The model under review builds one solid part; all positions refer to its coordinate system, in mm. Give positions to 0.01 mm unless a question says otherwise; leave off trailing zeros. Write each loop counter-clockwise with the first axis right and the second up, starting at its lowest first coordinate (ties: lowest second). Pieces come first, ordered by that corner, then holes. Notation, with made-up numbers: (-8.75, 35) -> (9.25, 35) arc R17 cw to (9.25, 48) -> close; hole circle Ø7 at (-1, 34.5). An arc over 180 degrees is marked (long way). Use CSV: the item, a comma, the result in double quotes.
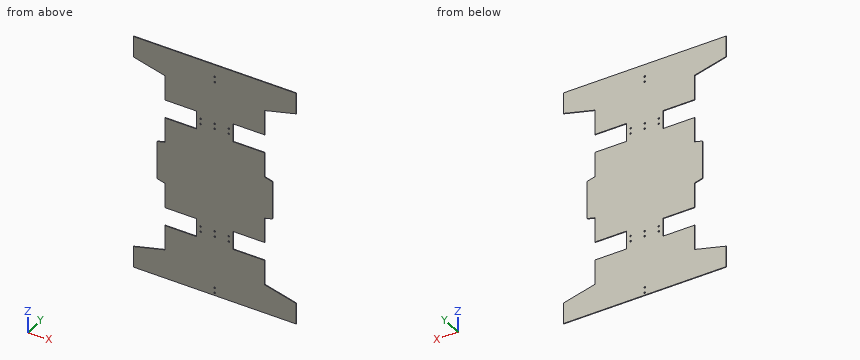
Autodesk Inventor part; units mm, degrees
ref_plane "YZ Plane" through (0, 0, 0) normal (1, 0, 0) x (0, 1, 0)
ref_plane "XZ Plane" through (0, 0, 0) normal (0, 1, 0) x (-1, 0, 0)
ref_plane "XY Plane" through (0, 0, 0) normal (0, 0, 1) x (1, 0, 0)
sketch "Sketch1" plane through (0, 0, 0) normal (0, 1, 0) x (-1, 0, 0)
  line L0 (359.9997, -324.9998) -> (359.9997, -389.9998)
  line L1 (359.9997, -389.9998) -> (239.9998, -420.0002)
  line L2 (359.9997, -194.9998) -> (359.9997, -129.9998)
  line L3 (359.9997, -129.9998) -> (239.9997, -99.9998)
  line L4 (359.9998, -615.0001) -> (359.9998, -550.0001)
  line L5 (359.9998, -550.0001) -> (239.9998, -520.0001)
  line L6 (359.9998, -745.0001) -> (359.9998, -810.0001)
  line L7 (359.9998, -810.0001) -> (239.9998, -840.0001)
  line L8 (740, -325.0005) -> (740, -390.0005)
  line L9 (740, -390.0005) -> (860, -420.0005)
  line L10 (740, -195.0005) -> (740, -130.0005)
  line L11 (740, -130.0005) -> (860, -100.0005)
  line L12 (740, -615.0001) -> (740, -550.0005)
  line L13 (740, -550.0005) -> (860, -520.0005)
  line L14 (740, -744.9998) -> (740, -809.9998)
  line L15 (740, -809.9998) -> (860, -839.9998)
  line L16 (860, -100.0005) -> (860, -19.9997)
  line L17 (860, -839.9998) -> (860, -919.9998)
  line L18 (239.9997, -99.9998) -> (239.9997, -19.9997)
  line L19 (239.9998, -840.0001) -> (239.9998, -920.0001)
  line L20 (859.9998, -19.9997) -> (379.9998, -19.9997)
  line L21 (860, -19.9997) -> (379.9998, -19.9997)
  line L22 (479.9997, -19.9997) -> (239.9997, -19.9997)
  line L23 (860, -919.9998) -> (139.9998, -919.9998)
  line L24 (239.9997, -19.9997) -> (859.9998, -19.9997)
  line L25 (860, -520.0005) -> (860, -420.0005)
  line L26 (239.9998, -520.0001) -> (239.9998, -420.0002)
  line L27 (479.9998, -744.9997) -> (479.9998, -745.0001)
  line L28 (479.9998, -745.0001) -> (479.9998, -615.0001)
  line L29 (479.9998, -615.0001) -> (359.9998, -615.0001)
  line L30 (479.9998, -745.0001) -> (359.9998, -745.0001)
  line L31 (620, -679.9998) -> (620, -745.0001)
  line L32 (620, -745.0001) -> (740, -744.9998)
  line L33 (620, -679.9998) -> (620, -615.0001)
  line L34 (740, -615.0001) -> (620, -615.0001)
  line L35 (620, -260.0005) -> (620, -325.0005)
  line L36 (620, -325.0005) -> (620, -195.0005)
  line L37 (620, -195.0005) -> (740, -195.0005)
  line L38 (620, -325.0005) -> (740, -325.0005)
  line L39 (479.9997, -260.0005) -> (479.9993, -325.0005)
  line L40 (479.9993, -325.0005) -> (359.9997, -324.9998)
  line L41 (479.9997, -260.0005) -> (479.9997, -195.0005)
  line L42 (479.9997, -195.0005) -> (359.9997, -194.9998)
  point P0 (479.9997, -19.9997)
  point P1 (740, -810.0001)
  point P2 (740, -550.0001)
  point P3 (740, -390.0001)
  point P4 (740, -130.0001)
  point P5 (239.9998, -919.9998)
  point P6 (239.9998, -919.9998)
  dimension "d44" = 0.45
  dimension "d16" = 80
  dimension "d23" = 65
extrude "Extrusion1" add sketch "Sketch1" along normal blind 3
sketch "Sketch2" plane through (0, 3, 0) normal (0, 1, 0) x (1, 0, 0)
  line L0 (-620, 325.0005) -> (-620, 195.0005)
  line L1 (-620, 260.0005) -> (-620, 225.0005)
  line L2 (-620, 225.0005) -> (-740, 225.0005)
  line L3 (-740, 195.0005) -> (-740, 130.0005)
  line L4 (-740, 225.0005) -> (-740, 195.0005)
  line L5 (-620, 260.0005) -> (-620, 295.0005)
  line L6 (-620, 295.0005) -> (-740, 295.0005)
  line L7 (-740, 295.0005) -> (-740, 325.0005)
  line L8 (-740, 325.0005) -> (-620, 325.0005)
  line L9 (-740, 325.0005) -> (-620, 325.0005)
  line L10 (-620, 325.0005) -> (-620, 295.0005)
  line L11 (-620, 225.0005) -> (-620, 195.0005)
  line L12 (-620, 195.0005) -> (-740, 195.0005)
  line L13 (-479.9997, 195.0005) -> (-479.9997, 260.0005)
  line L14 (-359.9997, 194.9998) -> (-479.9997, 195.0005)
  line L15 (-479.9997, 195.0005) -> (-359.9997, 194.9998)
  line L16 (-359.9997, 194.9998) -> (-359.9995, 225.0005)
  line L17 (-359.9995, 225.0005) -> (-479.9995, 225.0012)
  line L18 (-479.9995, 225.0012) -> (-479.9995, 295.0005)
  line L19 (-479.9997, 260.0005) -> (-479.9993, 325.0005)
  line L20 (-479.9993, 325.0005) -> (-359.9997, 324.9998)
  line L21 (-479.9993, 325.0005) -> (-359.9997, 324.9998)
  line L22 (-359.9997, 324.9998) -> (-359.9991, 295.0005)
  line L23 (-479.9995, 295.0005) -> (-359.9991, 295.0005)
  line L24 (-620, 745.0001) -> (-620, 615.0001)
  line L25 (-620, 680.0001) -> (-620, 645.0001)
  line L26 (-620, 645.0001) -> (-740, 645.0001)
  line L27 (-740, 645.0001) -> (-740, 615.0001)
  line L28 (-740, 615.0001) -> (-620, 615.0001)
  line L29 (-620, 615.0001) -> (-620, 645.0001)
  line L30 (-620, 680.0001) -> (-620, 715.0001)
  line L31 (-620, 715.0001) -> (-740, 715.0001)
  line L32 (-740, 744.9998) -> (-620, 745.0001)
  line L33 (-740, 715.0001) -> (-740, 744.9998)
  line L34 (-740, 744.9998) -> (-620, 745.0001)
  line L35 (-620, 745.0001) -> (-620, 715.0001)
  line L36 (-479.9998, 615.0001) -> (-479.9998, 745.0001)
  line L37 (-479.9998, 680.0001) -> (-479.9998, 645.0001)
  line L38 (-479.9998, 645.0001) -> (-359.9998, 645.0001)
  line L39 (-359.9998, 615.0001) -> (-479.9998, 615.0001)
  line L40 (-359.9998, 645.0001) -> (-359.9998, 615.0001)
  line L41 (-359.9998, 615.0001) -> (-479.9998, 615.0001)
  line L42 (-479.9998, 615.0001) -> (-479.9998, 645.0001)
  line L43 (-479.9998, 680.0001) -> (-479.9998, 715.0001)
  line L44 (-479.9998, 715.0001) -> (-359.9998, 715.0001)
  line L45 (-479.9998, 745.0001) -> (-359.9998, 745.0001)
  line L46 (-359.9998, 715.0001) -> (-359.9998, 745.0001)
  line L47 (-359.9998, 745.0001) -> (-479.9998, 745.0001)
  line L48 (-479.9998, 745.0001) -> (-479.9998, 715.0001)
  point P0 (0, 0)
  dimension "d26" = 35
  dimension "d27" = 35
  dimension "d28" = 35
  dimension "d29" = 35
  dimension "d30" = 35
  dimension "d31" = 35
extrude "Extrusion2" add sketch "Sketch2" against normal up to surface (3 mm away)
sketch "Sketch3" plane through (0, 3, 0) normal (0, 1, 0) x (1, 0, 0)
  line L0 (-620, 295.0005) -> (-620, 225.0005)
  line L1 (-620, 260.0005) -> (-620, 240.0005)
  line L2 (-620, 240.0005) -> (-479.9995, 240.0005)
  line L3 (-479.9995, 225.0012) -> (-479.9995, 295.0005)
  line L4 (-479.9995, 240.0005) -> (-479.9995, 280.0005)
  line L5 (-479.9995, 280.0005) -> (-620, 280.0005)
  line L6 (-620, 280.0005) -> (-620, 260.0005)
  line L7 (-620, 715.0001) -> (-620, 645.0001)
  line L8 (-620, 680.0001) -> (-620, 660.0001)
  line L9 (-620, 660.0001) -> (-479.9998, 660.0001)
  line L10 (-479.9998, 645.0001) -> (-479.9998, 715.0001)
  line L11 (-479.9998, 660.0001) -> (-479.9998, 680.0001)
  line L12 (-479.9998, 680.0001) -> (-479.9998, 700.0001)
  line L13 (-479.9998, 700.0001) -> (-620, 700.0001)
  line L14 (-620, 700.0001) -> (-620, 680.0001)
  point P0 (0, 0)
  dimension "d34" = 20
  dimension "d35" = 40
  dimension "d36" = 20
  dimension "d37" = 20
  dimension "d38" = 20
sketch "Sketch4" plane through (0, 3, 0) normal (0, 1, 0) x (1, 0, 0)
  line L0 (-860, 520.0005) -> (-860, 420.0005)
  line L1 (-860, 470.0005) -> (-828.2194, 470.0005)
  line L2 (-239.9998, 420.0002) -> (-239.9998, 520.0001)
  line L3 (-860, 19.9997) -> (-239.9997, 19.9997)
  line L4 (-549.9999, 19.9997) -> (-549.9999, 470.0003)
  line L5 (-549.9999, 470.0003) -> (-549.5499, 470.0003)
  line L6 (-549.9999, 470.0003) -> (-550.4499, 470.0003)
  circle A0 centre (-549.5499, 470.0003) radius 73.409
  point P0 (0, 0)
  dimension "d44" = 0.45
sketch "Sketch7" plane through (0, 3, 0) normal (0, 1, 0) x (1, 0, 0)
  circle A0 centre (-550, 66.9997) radius 3.05
  circle A1 centre (-550, 250.0005) radius 5
  circle A2 centre (-603.85, 270.0005) radius 4.6
  circle A3 centre (-603.85, 250.0005) radius 4.6
  circle A4 centre (-496.15, 250.0005) radius 5
  circle A5 centre (-496.15, 270.0005) radius 5
  line L0 (-537.75, 919.9998) -> (-562.25, 919.9998)
  line L1 (-537.75, 879.9998) -> (-537.75, 919.9998)
  line L2 (-562.25, 879.9998) -> (-537.75, 879.9998)
  line L3 (-562.25, 879.9998) -> (-562.25, 919.9998)
  circle A6 centre (-603.85, 690.0001) radius 4.6
  circle A7 centre (-603.85, 670.0001) radius 4.6
  circle A8 centre (-550, 690.0001) radius 4.6
  circle A9 centre (-550, 670.0001) radius 4.6
  circle A10 centre (-496.15, 690.0001) radius 4.6
  circle A11 centre (-496.15, 670.0001) radius 4.6
  circle A12 centre (-550, 66.9997) radius 3
  circle A13 centre (-550, 86.9997) radius 3
  circle A14 centre (-496.15, 250.0005) radius 3
  circle A15 centre (-496.15, 270.0005) radius 3
  circle A16 centre (-550, 250.0005) radius 3
  circle A17 centre (-550, 270.0005) radius 3
  circle A18 centre (-603.85, 250.0005) radius 3
  circle A19 centre (-603.85, 270.0005) radius 3
  circle A20 centre (-496.15, 670.0001) radius 3
  circle A21 centre (-496.15, 690.0001) radius 3
  circle A22 centre (-550, 670.0001) radius 3
  circle A23 centre (-550, 690.0001) radius 3
  circle A24 centre (-603.85, 670.0001) radius 3
  circle A25 centre (-603.85, 690.0001) radius 3
  circle A26 centre (-550, 889.9998) radius 3
  circle A27 centre (-550, 909.9998) radius 3
  point P0 (0, 0)
  dimension "d53" = 6
  dimension "d54" = 6
  dimension "d55" = 6
  dimension "d56" = 6
  dimension "d57" = 6
  dimension "d58" = 6
  dimension "d59" = 6
  dimension "d60" = 6
  dimension "d61" = 6
  dimension "d62" = 6
  dimension "d63" = 6
  dimension "d64" = 6
  dimension "d65" = 6
  dimension "d66" = 6
  dimension "d67" = 6
  dimension "d68" = 6
extrude "Extrusion7" cut sketch "Sketch7" against normal up to surface (3 mm away) contours A12 | A13 | A14 | A15 | A16 | A17 | A18 | A19 | A20 | A21 | A22 | A23 | A24 | A25 | A26 | A27
sketch "Sketch8" plane through (0, 3, 0) normal (0, 1, 0) x (1, 0, 0)
  line L0 (-239.9998, 420.0002) -> (-239.9998, 520.0001)
  line L1 (-860, 520.0005) -> (-860, 420.0005)
  line L2 (-769.488, 470.0005) -> (-769.488, 542.6285)
  line L3 (-740, 550.0005) -> (-860, 520.0005)
  line L4 (-769.488, 470.0005) -> (-769.488, 397.3725)
  line L5 (-860, 420.0005) -> (-740, 390.0005)
  line L6 (-330.5118, 470.0001) -> (-330.5118, 542.6281)
  line L7 (-239.9998, 520.0001) -> (-359.9998, 550.0001)
  line L8 (-330.5118, 470.0001) -> (-330.5118, 397.3719)
  line L9 (-359.9997, 389.9998) -> (-239.9998, 420.0002)
  point P0 (0, 0)
extrude "Extrusion8" cut sketch "Sketch8" against normal up to surface (3 mm away)
properties part number "base"
Q1. To check wall thickness, follow probe 1 along Z at (x, y) = (-463, 0.35); probe 2 along Z at (x, y) = (-603.85, 0.9); probe 3 along X at (y, z) = (1.5, -647). State the ranges of each line that lie inside material, in increasing order.
Derived:
probe 1,"z = -920 to -715, -645 to -295, -225 to -20"
probe 2,"z = -920 to -693, -687 to -673, -667 to -273, -267 to -253, -247 to -20"
probe 3,"x = -620 to -480"
Q2. Insertion check: pin 1 (1.5 mm diameter, centred on y = 1.5, z = -505, fed in from -X); pin 2 (1.5 mm diameter, centred on y = 1.5, z = -676, fed in from -X); pin 3 (1.5 mm diameter, centred on y = 1.5, z = -173.5, fed in from +X). Each pin has a flat end and moves straight along its axis. Give the tip position at first contact, or say it passes through.
Derived:
pin 1,"stops at x = -769.49"
pin 2,"stops at x = -620"
pin 3,"stops at x = -360"
Q3. Consider section B-B (x = -790). Write out the cut boundary in (y, z), then the cut area to 3 significant figures.
Derived:
outline,"(0, -920) -> (3, -920) -> (3, -822.5) -> (0, -822.5) -> close; (0, -117.5) -> (3, -117.5) -> (3, -20) -> (0, -20) -> close"
area,"585 mm2"
Q4. Consider section A-A (x = -703). Write out the cut boundary in (y, z), then the cut area to 3 significant figures.
Derived:
outline,"(0, -920) -> (3, -920) -> (3, -715) -> (0, -715) -> close; (0, -645) -> (3, -645) -> (3, -295) -> (0, -295) -> close; (0, -225) -> (3, -225) -> (3, -20) -> (0, -20) -> close"
area,"2,280 mm2"
Q5. Consider section C-C (z = -425.5). Write out the cut boundary in (x, y), then the cut area to 3 significant figures.
Derived:
outline,"(-769.49, 0) -> (-330.51, 0) -> (-330.51, 3) -> (-769.49, 3) -> close"
area,"1,320 mm2"
